Can you work these out from the model? Positions are in its coordinate system, mm. A direction names the side the tool comes from. Coordinates: 2 decimals unless noted, no trailing zeros. Loops run counter-clockwise (first coordinate to the right, second up) from the corner with the lowest first, then second, coordinate; pieces in that order, holes last.
```python
from build123d import *

# Parameters (mm, degrees)
ESQUISSE1_W                     = 50
ESQUISSE1_H                     = 48
BOSS_EXTRU_1_DEPTH              = 5
ESQUISSE2_R                     = 3
ESQUISSE2_R_2                   = 1.5
BOSS_EXTRU_2_DEPTH              = 3
R_P_TITION_LIN_AIRE1_COUNT      = 2
R_P_TITION_LIN_AIRE1_PITCH      = 21
R_P_TITION_LIN_AIRE1_COUNT_DIR2 = 2
R_P_TITION_LIN_AIRE1_PITCH_DIR2 = 12.5
ESQUISSE4_W                     = 6
ESQUISSE4_H                     = 5
BOSS_EXTRU_3_DEPTH              = 4
ESQUISSE5_R                     = 7
BOSS_EXTRU_4_DEPTH              = 6
ESQUISSE6_R                     = 1.75
ENL_V_MAT_EXTRU_1_DEPTH         = 6
ESQUISSE7_W                     = 50
ESQUISSE7_H                     = 10.758119029
ENL_V_MAT_EXTRU_2_DEPTH         = 10
CONG_2_R                        = 5
CONG_3_R                        = 3
ESQUISSE9_R                     = 1.5
ENL_V_MAT_EXTRU_3_DEPTH         = 70.161233188
ESQUISSE10_W                    = 22
ESQUISSE10_H                    = 5
ENL_V_MAT_EXTRU_4_DEPTH         = 10
ESQUISSE11_R                    = 3
BOSS_EXTRU_5_DEPTH              = 3
ESQUISSE12_R                    = 1.5
ENL_V_MAT_EXTRU_5_DEPTH         = 68.522412398


with BuildPart() as part:
    # Esquisse1 → Boss.-Extru.1 (new body)
    with BuildSketch(Plane.XY):
        with Locations((13.877005348, -12.235294118)):
            Rectangle(ESQUISSE1_W, ESQUISSE1_H)
    extrude(amount=BOSS_EXTRU_1_DEPTH)

    # Esquisse2 → Boss.-Extru.2 (add)
    with BuildSketch(Plane.XY.offset(5)):
        with Locations((3.377005348, -5.985294118)):
            Circle(ESQUISSE2_R)
        with Locations((3.377005348, -5.985294118)):
            Circle(ESQUISSE2_R_2, mode=Mode.SUBTRACT)
    boss_extru_2 = extrude(amount=BOSS_EXTRU_2_DEPTH)

    # Répétition linéaire1: Boss.-Extru.2 2 × 2
    with Locations(*[(i * R_P_TITION_LIN_AIRE1_PITCH, -j * R_P_TITION_LIN_AIRE1_PITCH_DIR2, 0) for i in range(R_P_TITION_LIN_AIRE1_COUNT) for j in range(R_P_TITION_LIN_AIRE1_COUNT_DIR2) if (i, j) != (0, 0)]):
        add(boss_extru_2)

    # Esquisse4 → Boss.-Extru.3 (add)
    with BuildSketch(Plane(origin=(0, -36.235294118, 0), x_dir=(-1, 0, 0), z_dir=(0, -1, 0))):
        with Locations((-13.877005348, -2.5)):
            Rectangle(ESQUISSE4_W, ESQUISSE4_H)
    extrude(amount=BOSS_EXTRU_3_DEPTH)

    # Esquisse5 → Boss.-Extru.4 (add)
    with BuildSketch(Plane.ZY.offset(-10.877005348)):
        with Locations((2.5, -46.773642533)):
            Circle(ESQUISSE5_R)
    extrude(amount=-BOSS_EXTRU_4_DEPTH)

    # Esquisse6 → Enlèv. mat.-Extru.1 (cut)
    with BuildSketch(Plane.ZY.offset(-10.877005348)):
        with Locations((2.5, -46.773642533)):
            Circle(ESQUISSE6_R)
    extrude(amount=-ENL_V_MAT_EXTRU_1_DEPTH, mode=Mode.SUBTRACT)

    # Esquisse7 → Enlèv. mat.-Extru.2 (cut)
    with BuildSketch(Plane.XY.offset(5)):
        with Locations((13.877005348, 6.385646368)):
            Rectangle(ESQUISSE7_W, ESQUISSE7_H)
    extrude(amount=-ENL_V_MAT_EXTRU_2_DEPTH, mode=Mode.SUBTRACT)

    # Congé2
    cong_2_edges = [part.edges().sort_by_distance(p)[0] for p in [
        (38.877005348, 1.006586853, 2.5),
        (-11.122994652, 1.006586853, 2.5),
        (38.877005348, -36.235294118, 2.5),
        (-11.122994652, -36.235294118, 2.5),
    ]]
    fillet(cong_2_edges, radius=CONG_2_R)

    # Congé3
    cong_3_edges = [part.edges().sort_by_distance(p)[0] for p in [
        (16.877005348, -36.235294118, 2.5),
        (10.877005348, -36.235294118, 2.5),
    ]]
    fillet(cong_3_edges, radius=CONG_3_R)

    # Esquisse9 → Enlèv. mat.-Extru.3 (cut, through all)
    with BuildSketch(Plane.XY.offset(15)):
        with Locations((3.377005348, -5.985294118)):
            Circle(ESQUISSE9_R)
        with Locations((24.377005348, -5.985294118)):
            Circle(ESQUISSE9_R)
        with Locations((24.377005348, -18.485294118)):
            Circle(ESQUISSE9_R)
        with Locations((3.377005348, -18.485294118)):
            Circle(ESQUISSE9_R)
    extrude(amount=-ENL_V_MAT_EXTRU_3_DEPTH, mode=Mode.SUBTRACT)

    # Esquisse10 → Enlèv. mat.-Extru.4 (cut)
    with BuildSketch(Plane.XY.offset(5)):
        with Locations((13.877005348, -28.735294118)):
            Rectangle(ESQUISSE10_W, ESQUISSE10_H)
    extrude(amount=-ENL_V_MAT_EXTRU_4_DEPTH, mode=Mode.SUBTRACT)

    # Esquisse11 → Boss.-Extru.5 (add)
    with BuildSketch(Plane(origin=(0, 0, 0), x_dir=(-1, 0, 0), z_dir=(0, 0, -1))):
        with Locations(Location((-21.877005348, -11.235294118, 0), (0, 0, 180))):
            Circle(ESQUISSE11_R)
        with Locations(Location((-5.877005348, -11.235294118, 0), (0, 0, 180))):
            Circle(ESQUISSE11_R)
    extrude(amount=BOSS_EXTRU_5_DEPTH)

    # Esquisse12 → Enlèv. mat.-Extru.5 (cut, through all)
    with BuildSketch(Plane(origin=(0, 0, -3), x_dir=(-1, 0, 0), z_dir=(0, 0, -1))):
        with Locations((-21.877005348, -11.235294118)):
            Circle(ESQUISSE12_R)
        with Locations((-5.877005348, -11.235294118)):
            Circle(ESQUISSE12_R)
    extrude(amount=-ENL_V_MAT_EXTRU_5_DEPTH, mode=Mode.SUBTRACT)


solid = part.part
```
(1) If I drill on probe 1 along X at (y, z) = (-18.5, 6.5); probe 2 along X at (y, z) = (-26.5, 3); probe 3 along Z at (x, y) = (12.5, -47), over which ranges is the centre line in solid material (lowest first)?
Check values:
probe 1: x = 0.38 to 1.88, 4.88 to 6.38, 21.38 to 22.88, 25.88 to 27.38
probe 2: x = -11.12 to 2.88, 24.88 to 38.88
probe 3: z = -4.5 to 0.76, 4.24 to 9.5
(2) I want a section at C-C on x = -1.5. Write out the boundary of the cut face in (y, z), then the cut area to 3 significant figures.
Check values:
outline: (-36.24, 0) - (1.01, 0) - (1.01, 5) - (-36.24, 5) - close
area: 186 mm2
(3) Which directions (+Z, -Z, +X, -X, +Y, -Y) give clear straight access to the entire face, cutting with the end or side of a thin tool? Please do faces 5 (the cylindrical face through (13.84, -48.48, 2.12)), 6 (the cylindrical face through (27.15, -7.13, 6.48)), 7 (the flat face through (16.877, -48, 4)), 8 (the cylindrical face through (2.88, -11.37, -1.48)).
Check values:
face 5: +X, -X
face 6: +Z
face 7: +Z, -Z, +X, -Y
face 8: -Z
(4) I'm going to push flat-ended pins straight in: pin 1 (3 mm diameter, centred on x = 23.5, y = -7, fed in from +Z); pin 2 (5 mm diameter, centred on x = -3.5, z = 1, fed in from -Y); pin 3 (2 mm diameter, centred on x = 12.5, z = 4.5, fed in from -Y); pin 4 (2.5 mm diameter, centred on x = 21.88, y = -11.24, fed in from -Z). Where does each tip first touch, or does it pass through?
Check values:
pin 1: stops at z = 8
pin 2: stops at y = -36.24
pin 3: stops at y = -53.7
pin 4: passes through
(5) I want a section at B-B on z = 2.5. State how many separate pieces and enclosed holes the cut face has, then the cut area to 3 significant figures.
Check values:
separate pieces: 2
enclosed holes: 7
area: 1,780 mm2
(6) I want a section at D-D on y = -22.5. Write out the boundary of the cut face in (x, z).
Check values:
outline: (-11.12, 0) - (38.88, 0) - (38.88, 5) - (-11.12, 5) - close
(7) If we mould it in two halves opening along X, with no side actions, what happens to faces 1 (the flat face through (14, -26.235, 3)), 2 (the cylindrical face through (17.73, -37.14, 2.46)), 3 (the flat face through (2, -7, 8)), 4 (the cylindrical face through (24.05, -7.45, 4.06))? For each: released by +X, released by -X, zero draft, split by the parting line, or undercut.
Check values:
face 1: undercut
face 2: released by +X
face 3: zero draft
face 4: undercut
(8) I want a section at A-A on z = -1. Write out the boundary of the cut face in (x, y).
Check values:
outline: circle Ø6 at (5.88, -11.24); (10.88, -52.84) - (16.88, -52.84) - (16.88, -40.71) - (10.88, -40.71) - close; circle Ø6 at (21.88, -11.24); hole circle Ø3 at (5.88, -11.24); hole circle Ø3 at (21.88, -11.24)
